from build123d import *

# Parameters (mm, degrees)
BOSS_EXTRUDE1_DEPTH = 29.21
SKETCH2_W           = 21.206924152
SKETCH2_H           = 28.633723015
SKETCH2_R           = 3.175
BOSS_EXTRUDE2_DEPTH = 3.81
BOSS_EXTRUDE3_START = -4.826
SKETCH3_R           = 3.175
BOSS_EXTRUDE3_DEPTH = 4.826
SKETCH4_R           = 2.924709064
SKETCH4_R_2         = 3.042286042
BOSS_EXTRUDE4_DEPTH = 3.81


with BuildPart() as part:
    # Sketch1 → Boss-Extrude1 (new body)
    with BuildSketch(Plane.XY):
        with BuildLine():
            Line((92.017977945, 102.236000374), (113.224902097, 102.236000374))
            Line((113.224902097, 102.236000374), (113.210298678, 106.295173442))
            Line((113.210298678, 106.295173442), (104.041152894, 106.300000374))
            ThreePointArc((104.041152894, 106.300000374), (97.620882741, 109.755229578), (96.960558709, 117.016252224))
            ThreePointArc((96.960558709, 117.016252224), (97.366531104, 119.0035195), (96.962652269, 120.991213315))
            ThreePointArc((96.962652269, 120.991213315), (96.669783853, 126.656600471), (100.468728286, 130.869723389))
            Line((100.468728286, 130.869723389), (92.017977945, 130.869723389))
            Line((92.017977945, 130.869723389), (92.017977945, 102.236000374))
        make_face()
    extrude(amount=-BOSS_EXTRUDE1_DEPTH)

    # Sketch2 → Boss-Extrude2 (add)
    with BuildSketch(Plane.XY):
        with Locations((102.621440021, 116.552861882)):
            Rectangle(SKETCH2_W, SKETCH2_H)
        with Locations(Location((104.05047074, 124, 0), (0, 0, 180))):
            Circle(SKETCH2_R, mode=Mode.SUBTRACT)
        with Locations(Location((104.04520642, 114, 0), (0, 0, 180))):
            Circle(SKETCH2_R, mode=Mode.SUBTRACT)
    extrude(amount=BOSS_EXTRUDE2_DEPTH)

    # Sketch3 → Boss-Extrude3 (add)
    with BuildSketch(Plane(origin=(0, 0, -29.21), x_dir=(-1, 0, 0), z_dir=(0, 0, -1)).offset(BOSS_EXTRUDE3_START)):
        with BuildLine():
            Line((-113.210298678, 106.295173442), (-113.210298678, 130.994991711))
            Line((-113.210298678, 130.994991711), (-100.468728286, 130.869723389))
            ThreePointArc((-100.468728286, 130.869723389), (-96.669783853, 126.656600471), (-96.962652269, 120.991213315))
            ThreePointArc((-96.962652269, 120.991213315), (-97.366531104, 119.0035195), (-96.960558709, 117.016252224))
            ThreePointArc((-96.960558709, 117.016252224), (-97.620882741, 109.755229578), (-104.041152894, 106.300000374))
            Line((-104.041152894, 106.300000374), (-113.210298678, 106.295173442))
        make_face()
        with Locations((-104.04520642, 114)):
            Circle(SKETCH3_R, mode=Mode.SUBTRACT)
        with Locations((-104.05047074, 124)):
            Circle(SKETCH3_R, mode=Mode.SUBTRACT)
    extrude(amount=BOSS_EXTRUDE3_DEPTH)

    # Sketch4 → Boss-Extrude4 (add)
    with BuildSketch(Plane(origin=(0, 102.236000374, 0), x_dir=(1, 0, 0), z_dir=(0, 1, 0))):
        Polygon((92.017977945, -3.81), (92.017977945, -30.273157469), (113.224902097, -30.273157469), (113.224902097, -3.81), (113.224902097, 29.21), (102.326996441, 52.536371302), (80.454002019, 52.536371302), (92.017977945, 29.21), align=None)
        with Locations(Location((96.881668056, 40.935379723, 0), (0, 0, 270))):
            Circle(SKETCH4_R, mode=Mode.SUBTRACT)
        with Locations(Location((102.326996441, -18.162627323, 0), (0, 0, 270))):
            Circle(SKETCH4_R_2, mode=Mode.SUBTRACT)
    extrude(amount=-BOSS_EXTRUDE4_DEPTH)


solid = part.part
Model file for the job. Use its own axes, mm. A direction names the side the tool comes from. Give positions to 0.01 mm unless a question says otherwise; leave off trailing zeros. Order: outer loops, then holes, each group sorted by start corner. A loop starts at its lowest first (then second) coordinate and runs counter-clockwise, first axis right, second up. Notation, with made-up numbers: (21.25, 16.5) - (47.25, 16.5) arc R35 ccw to (47.25, 50.5) - close; hole circle Ø2 at (84.5, 10.5). An arc over 180 degrees is marked (long way). One line per item, written item: value.
Item 1: Slice it at C-C (y = 124). List the corners of the cut face in (x, z) (3 decimals).
Response values:
outline: (92.018, -29.21) - (100.875, -29.21) - (100.875, -24.384) - (96.245, -24.384) - (96.245, 0) - (100.875, 0) - (100.875, 3.81) - (92.018, 3.81) - close; (107.225, -29.21) - (113.21, -29.21) - (113.21, -24.384) - (107.225, -24.384) - close; (107.225, 0) - (113.225, 0) - (113.225, 3.81) - (107.225, 3.81) - close
Item 2: Pin check, flat tips, straight feed: pin 1 Ø12 at (y, z) = (115, 0.5) entering from -X; pin 2 Ø10 at (x, y) = (104.05, 114) entering from -Z; pin 3 Ø18.5 at (x, z) = (92, -41) entering from +Y. Stop position of each tip, or through.
Response values:
pin 1: x = 92.02
pin 2: z = -29.21
pin 3: y = 102.24
Item 3: Slice it at A-A (z = -41.5). List the corners of the cut face in (x, y), then the cut area to 3 significant figures.
Response values:
outline: (85.93, 98.43) - (94.01, 98.43) - (94.01, 102.24) - (85.93, 102.24) - close; (99.75, 98.43) - (107.48, 98.43) - (107.48, 102.24) - (99.75, 102.24) - close
area: 60.3 mm2
Item 4: Slice it at D-D (z = -16.5). List the corners of the cut face in (x, y), then the cut area to 3 significant figures.
Response values:
outline: (92.02, 98.43) - (113.22, 98.43) - (113.22, 102.24) - (113.21, 106.3) - (104.04, 106.3) arc R7.7 cw to (96.96, 117.02) arc R5.08 ccw to (96.96, 120.99) arc R7.41 cw to (100.47, 130.87) - (92.02, 130.87) - close
area: 298 mm2
Item 5: Wall check: line 1 (Z direction, x = 111.5, y = 124.5); line 2 (X direction, y = 124, z = 1.75); line 3 (X direction, y = 118.5, z = 1.5). Give the ranges that are in metal, low to high.
Response values:
line 1: -29.21 to -24.38, 0 to 3.81
line 2: 92.02 to 100.88, 107.23 to 113.22
line 3: 92.02 to 113.22
Item 6: Two-plate mould, pull along Y, no slides. Class faces 1 (the flat face through (102, 117, -29.21)), 2 (the cylindrical face through (97.68, 109.67, -12.02)), 3 (the flat face through (100, 98.426, -12)), 4 (the flat face through (102, 102.236, 14)): released by +Y, released by -Y, zero draft, split by the parting line, or undercut.
Response values:
face 1: zero draft
face 2: undercut
face 3: released by -Y
face 4: released by +Y
Item 7: Tool access for faces 5 (the flat face through (92.018, 115, -13)), 6 (the cylindrical face through (99.357, 100.358, 17.503)), 7 (the flat face through (105, 119, -24.384)), 8 (the flat face through (100, 117, 3.81)): list every direction of +Z, -Z, +X, -X, +Y, -Y with a clear straight run to the whole face (end or side of a thin tool).
Response values:
face 5: +Z, -X, +Y, -Y
face 6: +Y, -Y
face 7: +X
face 8: +Z, +X, -X, +Y
Item 8: Slice it at B-B (y = 114). List the corners of the cut face in (x, z), then the cut area to 3 significant figures.
Response values:
outline: (92.02, -29.21) - (100.87, -29.21) - (100.87, -24.38) - (96.35, -24.38) - (96.35, 0) - (100.87, 0) - (100.87, 3.81) - (92.02, 3.81) - close; (107.22, -29.21) - (113.21, -29.21) - (113.21, -24.38) - (107.22, -24.38) - close; (107.22, 0) - (113.22, 0) - (113.22, 3.81) - (107.22, 3.81) - close
area: 234 mm2
